```python
from build123d import *

# Parameters (mm, degrees)
SKETCH1_R           = 4
BOSS_EXTRUDE1_DEPTH = 18
SKETCH2_R           = 4.5
CUT_EXTRUDE1_DEPTH  = 61.218975205


with BuildPart() as part:
    # Sketch1 → Boss-Extrude1 (new body)
    with BuildSketch(Plane(origin=(0, 0, 0), x_dir=(0, 0, -1), z_dir=(1, 0, 0))):
        Polygon((-11.25, 23.75), (15.939233611, 36.428547852), (29.376155741, 7.612975355), (11.25, -0.83938988), (11.25, -23.75), (-11.25, -23.75), align=None)
        with Locations((0, -14.75)):
            Circle(SKETCH1_R, mode=Mode.SUBTRACT)
        with Locations((0, 5.25)):
            Circle(SKETCH1_R, mode=Mode.SUBTRACT)
    extrude(amount=BOSS_EXTRUDE1_DEPTH)

    # Sketch2 → Cut-Extrude1 (cut, through all)
    with BuildSketch(Plane(origin=(0, 23.817102858, 11.106097458), x_dir=(1, 0, 0), z_dir=(0, 0.906307787, 0.422618262))):
        with Locations((8, 19.841221112)):
            Circle(SKETCH2_R)
    extrude(amount=-CUT_EXTRUDE1_DEPTH, mode=Mode.SUBTRACT)


solid = part.part
```
Design review of the part built by this model. Coordinates are the model's own, in mm. A direction names the side the tool comes from. Coordinates: 2 decimals unless noted, no trailing zeros. Loops run counter-clockwise (first coordinate to the right, second up) from the corner with the lowest first, then second, coordinate; pieces in that order, holes last. Notation, with made-up numbers: M 64,23.5 L 121,23.5 A18 cw 121,56.5 Z; hole C 33,9.5 d6. An arc over 180 degrees is marked long. One line per question, with ' | ' between items.
(1) Machinability: for faces 5 (the face through (9, -23.75, 0)), 6 (the face through (9, -12, -11.25)), which of the approach directions +Z, -Z, +X, -X, +Y, -Y give a long, thin tool a straight path to every point of the face, cutting with its end or side? Answer none if there is none.
Filled in:
face 5: +Z, -Z, +X, -X, -Y | face 6: -Z, +X, -X, -Y
(2) We need section C-C (y = -14.75). Give the boundary of the cut face in (x, z), and give its area (3 significant figures).
Filled in:
outline: M 0,-11.25 L 18,-11.25 L 18,-4 L 0,-4 Z; M 0,4 L 18,4 L 18,11.25 L 0,11.25 Z | area: 261 mm^2
(3) For pin 1 Ø4 at (x, y) = (3.5, 16.5) entering from -Z; pin 2 Ø1 at (x, y) = (2, 4.5) entering from -Z, all flat-tipped, find the tip position at first contact; note any pin that passes through.
Filled in:
pin 1: stops at z = -26.16 | pin 2: stops at z = -23.77
(4) We need section B-B (z = 0). Give the boundary of the cut face in (x, y), and give its area (3 significant figures).
Filled in:
outline: M 0,-23.75 L 18,-23.75 L 18,-18.75 L 0,-18.75 Z; M 0,-10.75 L 18,-10.75 L 18,1.25 L 0,1.25 Z; M 0,9.25 L 18,9.25 L 18,29 L 0,29 Z | area: 661 mm^2
(5) Wall thickness on probe 1 along Y at (x, z) = (8, 0); probe 2 along Z at (x, y) = (1.75, -7.5); probe 3 along X at (y, z) = (15.5, -13.5): over which ranges is each line inside the solid? List them lowest first.
Filled in:
probe 1: y = -23.75 to -18.75, -10.75 to 1.25, 9.25 to 29 | probe 2: z = -11.25 to 11.25 | probe 3: x = 0 to 3.63, 12.37 to 18
(6) We need section D-D (x = 15.5). Give the boundary of the cut face in (y, z).
Filled in:
outline: M -23.75,-11.25 L -0.84,-11.25 L 7.61,-29.38 L 36.43,-15.94 L 23.75,11.25 L -23.75,11.25 Z; hole C -14.75,0 d8; hole C 5.25,0 d8
(7) Draft analysis for pull direction Z (two halves, no side actions). For faces 1 (the face through (8.87, 30, -2.15)), 2 (the face through (12.29, 18.57, -14.73)), 3 (the face through (8.9, -13.5, -3.8)), 4 (the face through (18, 7, -5)), state which applies: released by +Z, released by -Z, zero draft, split by the parting line, or undercut.
Filled in:
face 1: released by +Z | face 2: undercut | face 3: undercut | face 4: zero draft
(8) We need section A-A (x = 10.5). Give the boundary of the cut face in (y, z).
Filled in:
outline: M -23.75,-11.25 L -0.84,-11.25 L 1.81,-16.92 L 30.62,-3.49 L 23.75,11.25 L -23.75,11.25 Z; M 4.97,-23.7 L 7.61,-29.38 L 36.43,-15.94 L 33.78,-10.27 Z; hole C -14.75,0 d8; hole C 5.25,0 d8
